Part model, mm, in its own coordinate system. A direction names the side the tool comes from. Round coordinates to 2 decimals unless told otherwise and drop trailing zeros. Loops run counter-clockwise (first coordinate to the right, second up) from the corner with the lowest first, then second, coordinate; pieces in that order, holes last. Notation, with made-up numbers: M 22.5,-40 L 56.5,-40 A30 cw 56.5,-6 Z; hole C 53,51.25 d7. An arc over 180 degrees is marked long. Write each question's results on one line, items separated by ' | '.
Autodesk Inventor part; units mm, degrees
ref_plane "YZ Plane" through (0, 0, 0) normal (1, 0, 0) x (0, 1, 0)
ref_plane "XZ Plane" through (0, 0, 0) normal (0, 1, 0) x (-1, 0, 0)
ref_plane "XY Plane" through (0, 0, 0) normal (0, 0, 1) x (1, 0, 0)
sketch "Sketch1" plane through (0, 0, 0) normal (1, 0, 0) x (0, 1, 0)
  line L0 (0, 0) -> (0, -110)
  line L1 (0, -110) -> (3, -110)
  line L2 (3, -110) -> (3, 0)
  line L3 (3, 0) -> (0, 0)
  line L4 (3, 0) -> (3, -5)
  line L5 (3, -110) -> (3, -105)
  line L6 (3, -110) -> (5, -110)
  line L7 (5, -110) -> (5, -105)
  line L8 (5, -105) -> (3, -105)
  line L9 (3, 0) -> (5, 0)
  line L10 (5, 0) -> (5, -5)
  line L11 (5, -5) -> (3, -5)
  line L12 (3, -105) -> (1, -105)
  line L13 (1, -105) -> (1, -5)
  line L14 (1, -5) -> (3, -5)
  line L15 (5, -5) -> (5, -6)
  line L16 (5, -6) -> (1, -6)
  line L17 (5, -105) -> (5, -104)
  line L18 (5, -104) -> (1, -104)
  line L19 (3, -6) -> (3.1, -6)
  line L20 (2.5, -6) -> (2.5, -104)
  point P0 (3, -104)
  point P1 (2, -6)
  point P2 (3.1, -104)
  dimension "d0" = 110
  dimension "d1" = 3
  dimension "d2" = 5
  dimension "d3" = 5
  dimension "d5" = 2
  dimension "d6" = 2
  dimension "d7" = 2
  dimension "d8" = 1
  dimension "d9" = 1
  dimension "d22" = 1.5
revolve "Revolution1" add sketch "Sketch1" angle 360 about axis through (0, 0, 0) along (0, 0, -1) contours L9 L10 L11 L2 | L2 L8 L7 L6 | L11 L15 L16 L2 | L2 L16 L13 L14 | L12 L13 L18 L2 | L2 L18 L17 L8 | L20 L18 L13 L16
thread "Thread1"
thread "Thread2"
chamfer "Chamfer1" distance 0.5 angle 45 2 edges at (0, -3, 0) (0, -3, -110)
chamfer "Chamfer2" distance 0.5 angle 45 4 edges at (0, -5, -110) (0, -5, -104) (0, -5, -6) (0, -5, 0)
fillet "Fillet1" radius 2 2 edges at (0, -2.5, -104) (0, -2.5, -6)
properties part number "Heater"
Item 1: Band-saw the part on A-A on z = -69. Give the cut face in (x, y).
Filled sheet:
outline: C 0,0 d5; hole C 0,0 d2
Item 2: Wall check: L1, parallel to X at y = 0, z = -67.5; L2, parallel to X at y = 0, z = -106.3; L3, parallel to Z at x = 1, y = 3.75. Give the ranges that are in metal, low to high.
Filled sheet:
L1: -2.5 to -1, 1 to 2.5 | L2: -5 to -3, 3 to 5 | L3: -110 to -103.9, -6.1 to 0
Item 3: Which spindle directions (+Z, -Z, +X, -X, +Y, -Y) get a long thin tool onto all of the face, cutting with end or side? Do faces 1 (the flat face through (1, -1, -5)), 2 (the cylindrical face through (0, -3, -107)), 3 (the cylindrical face through (-2.44, -0.54, -55.66)). Say none if no direction does.
Filled sheet:
face 1: +Z | face 2: -Z | face 3: none
Item 4: Drop flat-ended pins along their axis: P1, Ø5, axis at x = 2.5, z = -55, coming from the -Y side; P2, Ø1, axis at x = 0, z = -27, coming from the +Y side; P3, Ø6, axis at y = -0.5, z = -59, coming from the -X side. Give the stop position or say it passes through.
Filled sheet:
P1: y = -2.5 | P2: y = 2.5 | P3: x = -2.5
Item 5: Two-plate mould, pull along Y, no slides. Class faces 4 (the cylindrical face through (1, 0, -54)), 5 (the cylindrical face through (-4.88, -1.08, -3.04)), 6 (the flat face through (-4, 0, 0)): +Y half, -Y half, draft (parallel to the pull), parting line (faces both ways), or undercut.
Filled sheet:
face 4: undercut | face 5: parting line | face 6: draft
